The model under review builds one solid part; all positions refer to its coordinate system, in mm. A direction names the side the tool comes from. Round coordinates to 2 decimals unless told otherwise and drop trailing zeros. Order: outer loops, then holes, each group sorted by start corner. A loop starts at its lowest first (then second) coordinate and runs counter-clockwise, first axis right, second up. Notation, with made-up numbers: M 63.5,-32 L 94.5,-32 A15 cw 94.5,-22 Z; hole C -23.75,75.5 d2. An arc over 180 degrees is marked long. Answer as a JSON object with one key per item and string values. Group by question number.
1. Add section C-C on x = 0. State the section outline as (y, z) points, and give its area (3 significant figures).
2. Mouldability with a two-part tool opening along X and no side actions: class faces 1 (the face through (-0.08, 0.79, 7.43)), 2 (the face through (-8.382, 1, -20)), 3 (the face through (11.176, 1, 1)) as released by +X, released by -X, zero draft, split by the parting line, or undercut.
3. Add section B-B on y = 9.5. State the section outline as (x, z) points.
4. Machinability: for faces 4 (the face through (-2.54, 3, 3)), 5 (the face through (-1, 8, 2.35)), 6 (the face through (6.985, -1, -3)), which of the approach directions +Z, -Z, +X, -X, +Y, -Y give a long, thin tool a straight path to every point of the face, cutting with its end or side? Answer none if there is none.
5. Add section D-D on z = 10.5. State the section outline as (x, y) points.
6. To check wall thickness, follow probe 1 along Z at (x, y) = (0, 0.95); probe 2 along X at (y, z) = (-1, -3) (3 decimals); probe 3 along Y at (x, z) = (-2.75, 11). State the ranges of each line that lie inside material, in increasing order. Write a range as [from, to].
7. Clearance check with flat-ended pins moving along their axes: P1, Ø11, axis at x = -0.5, z = -13, coming from the +Y side; P2, Ø1, axis at x = -1, y = 3.5, coming from the +Z side; P3, Ø1.1, axis at y = 8.5, z = 0.5, coming from the -X side. State where each tip first meets the part, or that it passes through.
8. Add section A-A on y = -0.5. State the section outline as (x, z) points (1 decimal).
Autodesk Inventor part; units mm, degrees
ref_plane "YZ Plane" through (0, 0, 0) normal (1, 0, 0) x (0, 1, 0)
ref_plane "XZ Plane" through (0, 0, 0) normal (0, 1, 0) x (-1, 0, 0)
ref_plane "XY Plane" through (0, 0, 0) normal (0, 0, 1) x (1, 0, 0)
sketch "Sketch1" plane through (0, 0, 0) normal (0, 1, 0) x (-1, 0, 0)
  line L0 (11.176, 13.3985) -> (-11.176, 13.3985)
  line L1 (-11.176, 13.3985) -> (-11.176, -11.4935)
  line L2 (11.176, -11.4935) -> (11.176, 13.3985)
  line L3 (11.176, 13.3985) -> (-11.176, -13.3985) construction
  line L4 (0, 20.6375) -> (0, -33.0464)
  line L5 (-8.382, -13.3985) -> (-8.382, -26.8605)
  line L6 (-8.382, -26.8605) -> (8.382, -26.8605)
  line L7 (8.382, -26.8605) -> (8.382, -13.3985)
  line L8 (9.271, -13.3985) -> (11.176, -11.4935)
  line L9 (-9.271, -13.3985) -> (-11.176, -11.4935)
  line L10 (-9.271, -13.3985) -> (-8.382, -13.3985)
  line L11 (8.382, -13.3985) -> (9.271, -13.3985)
  point P0 (0, 0)
  point P1 (11.176, -13.3985)
  point P2 (0, 0)
  dimension "d0" = 22.352
  dimension "d1" = 26.797
  dimension "d2" = 16.764
  dimension "d3" = 13.462
  dimension "d4" = 1.905
  dimension "d5" = 1.905
  dimension "d6" = 1.905
  dimension "d7" = 1.905
extrude "Extrusion1" add sketch "Sketch1" along normal blind 1.6002
sketch "Sketch2" plane through (0, 1.6002, 0) normal (0, 1, 0) x (1, 0, 0)
  line L0 (-11.176, -13.3985) -> (11.176, -13.3985)
  line L1 (8.382, 26.8605) -> (-8.382, 26.8605)
  line L2 (0, -15.1574) -> (0, 42.0562)
  line L3 (0, -15.1574) -> (57.2136, -15.1574) construction
  point P0 (0, 0)
  point P1 (0, -9.1567)
  point P2 (0, 23.8887)
  dimension "d10" = 4.2418
  dimension "d11" = 2.9718
  dimension "d12" = 90
hole "Hole1" at (0, 1.6002, 9.1567) at (0, 1.6002, -23.8887) direction (0, -1, 0) diameter 3.4544 end through all
sketch "Sketch3" plane through (0, 1.6002, 0) normal (0, 1, 0) x (1, 0, 0)
  line L0 (-2.54, 0.9525) -> (2.54, 0.9525)
  line L1 (2.54, 0.9525) -> (2.54, -6.6675)
  line L2 (2.54, -6.6675) -> (-2.54, -6.6675)
  line L3 (-2.54, -6.6675) -> (-2.54, 0.9525)
  line L4 (0, 0) -> (0, 29.7759)
  line L5 (0, 0) -> (29.7759, 0) construction
  line L6 (0, 0) -> (0, -24.9457)
  line L7 (0, 0) -> (24.9457, 0) construction
  line L8 (-2.54, 0.9525) -> (2.54, -6.6675) construction
  line L9 (-11.176, -13.3985) -> (11.176, -13.3985) construction
  point P0 (0, -2.8575)
  dimension "d20" = 90
  dimension "d21" = 90
  dimension "d22" = 10.541
  dimension "d23" = 5.08
  dimension "d24" = 7.62
extrude "Extrusion2" add sketch "Sketch3" along normal blind 3.175
sketch "Sketch4" plane through (0, 4.7752, 0) normal (0, 1, 0) x (1, 0, 0)
  line L0 (0, 1.9235) -> (0, -7.9336)
  line L1 (-5.0807, -2.8575) -> (5.7317, -2.8575)
  line L2 (2.54, 0.9525) -> (-2.54, 0.9525)
  line L3 (2.54, -6.6675) -> (2.54, 0.9525)
  line L4 (-1.778, 0.1905) -> (-0.762, 0.1905)
  line L5 (-0.762, 0.1905) -> (-0.762, -0.8255)
  line L6 (-0.762, -0.8255) -> (-1.778, -0.8255)
  line L7 (-1.778, -0.8255) -> (-1.778, 0.1905)
  point P0 (0, 0)
  point P1 (0, 0.9525)
  point P2 (2.54, -2.8575)
  dimension "d27" = 1.016
  dimension "d28" = 1.016
  dimension "d29" = 1.524
  dimension "d30" = 4.064
extrude "Extrusion3" add sketch "Sketch4" along normal blind 5.9944 contours L4 L5 L6 L7
pattern_linear "Rectangular Pattern1" count 2 spacing 2.54 along (1, 0, 0) count 3 spacing 2.54 along (0, 0, 1) of "Extrusion3"
sketch "Sketch5" plane through (0, 0, 0) normal (0, -1, 0) x (1, 0, 0)
  line L0 (0, 15.1213) -> (0, -35.4386)
  line L1 (6.985, -1.5875) -> (4.318, -1.5875)
  line L2 (4.318, -1.5875) -> (4.318, -4.9403)
  line L3 (4.318, -4.9403) -> (6.985, -4.9403)
  line L4 (6.985, -4.9403) -> (6.985, -1.5875)
  line L5 (-11.176, 13.3985) -> (11.176, 13.3985)
  line L6 (-4.318, -4.9403) -> (-6.985, -4.9403)
  line L7 (-6.985, -4.9403) -> (-6.985, -1.5875)
  line L8 (-6.985, -1.5875) -> (-4.318, -1.5875)
  line L9 (-4.318, -1.5875) -> (-4.318, -4.9403)
  point P0 (0, 0)
  dimension "d39" = 2.667
  dimension "d40" = 3.3528
  dimension "d41" = 8.636
  dimension "d42" = 14.986
  dimension "d43" = 8.636
extrude "Extrusion4" add sketch "Sketch5" along normal blind 1.651
equation "\"d6\" = d4"
equation "\"d7\" = d6"
equation "\"d43\" = d41"
properties part number "wheel_encoder"
Recorded:
{
 "1": {"outline": "M 0,-26.86 L 1.6,-26.86 L 1.6,-25.62 L 0,-25.62 Z; M 0,-22.16 L 1.6,-22.16 L 1.6,-0.95 L 4.78,-0.95 L 4.78,6.67 L 1.6,6.67 L 1.6,7.43 L 0,7.43 Z; M 0,10.88 L 1.6,10.88 L 1.6,13.4 L 0,13.4 Z", "area": "77.6 mm²"},
 "2": {"face 1": "undercut", "face 2": "released by -X", "face 3": "released by +X"},
 "3": {"outline": "M -1.78,-0.19 L -0.76,-0.19 L -0.76,0.83 L -1.78,0.83 Z; M -1.78,2.35 L -0.76,2.35 L -0.76,3.37 L -1.78,3.37 Z; M -1.78,4.89 L -0.76,4.89 L -0.76,5.91 L -1.78,5.91 Z; M 0.76,-0.19 L 1.78,-0.19 L 1.78,0.83 L 0.76,0.83 Z; M 0.76,2.35 L 1.78,2.35 L 1.78,3.37 L 0.76,3.37 Z; M 0.76,4.89 L 1.78,4.89 L 1.78,5.91 L 0.76,5.91 Z"},
 "4": {"face 4": "+Z, -Z, -X, +Y", "face 5": "+X, -X, +Y", "face 6": "+Z, -Z, +X, -Y"},
 "5": {"outline": "M -11.18,0 L -1.09,0 L -1.09,1.6 L -11.18,1.6 Z; M 1.09,0 L 11.18,0 L 11.18,1.6 L 1.09,1.6 Z"},
 "6": {"probe 1": "z = [-26.86, -25.62], [-22.16, 7.43], [10.88, 13.4]", "probe 2": "x = [-6.985, -4.318], [4.318, 6.985]", "probe 3": "y = [0, 1.6]"},
 "7": {"P1": "stops at y = 1.6", "P2": "stops at z = 6.67", "P3": "stops at x = -1.78"},
 "8": {"outline": "M -7,-4.9 L -4.3,-4.9 L -4.3,-1.6 L -7,-1.6 Z; M 4.3,-4.9 L 7,-4.9 L 7,-1.6 L 4.3,-1.6 Z"}
}
